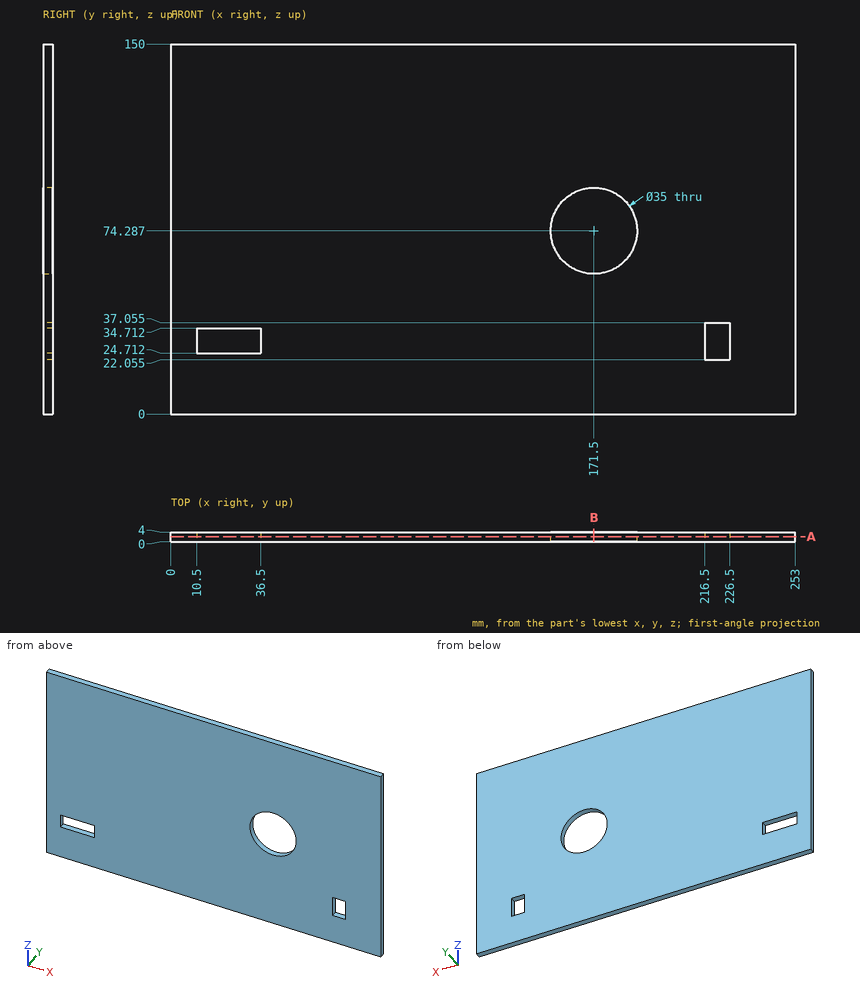
Part print with two shaded views. Sizes in mm from the minimum x, y, z corner. Round coordinates to 2 decimals unless told otherwise and drop trailing zeros. Write each loop counter-clockwise with the first axis right and the second up, starting at its lowest first coordinate (ties: lowest second). Pieces come first, ordered by that corner, then holes. Notation, with made-up numbers: (24.5, 58.5) -> (46.5, 58.5) arc R27 cw to (46.5, 96.5) -> close; hole circle Ø7 at (-5, -32.5). An arc over 180 degrees is marked (long way). Use one line per item in the form item = value.
Q1. Drill centre lines: L1, parallel to X at y = 3.6, z = 34; L2, parallel to Z at x = 31.5, y = 3.35; L3, parallel to X at y = 2.45, z = 82.5. Where is each one in solid material? Low to high.
Conclusion:
L1 = 0 to 10.5, 36.5 to 216.5, 226.5 to 253
L2 = 0 to 24.71, 34.71 to 150
L3 = 0 to 156.05, 186.95 to 253
Q2. Band-saw the part on B-B, the plane x = 171.5. Write the cut outline in (y, z), then the cut area to 3 significant figures.
Conclusion:
outline = (0, 0) -> (4, 0) -> (4, 56.79) -> (0, 56.79) -> close; (0, 91.79) -> (4, 91.79) -> (4, 150) -> (0, 150) -> close
area = 460 mm²
Q3. Band-saw the part on A-A, the plane y = 2.15. Write the cut outline in (x, z) (1 decimal).
Conclusion:
outline = (0, 0) -> (253, 0) -> (253, 150) -> (0, 150) -> close; hole (10.5, 24.7) -> (36.5, 24.7) -> (36.5, 34.7) -> (10.5, 34.7) -> close; hole circle Ø35 at (171.5, 74.3); hole (216.5, 22.1) -> (226.5, 22.1) -> (226.5, 37.1) -> (216.5, 37.1) -> close
